Here's how the part is built. I have some questions about the finished solid (model axes, mm). Face numbers are marked on the shaded views. A direction names the side the tool comes from. Round coordinates to 2 decimals unless told otherwise and drop trailing zeros. Order: outer loops, then holes, each group sorted by start corner. A loop starts at its lowest first (then second) coordinate and runs counter-clockwise, first axis right, second up. Notation, with made-up numbers: (-21.5, 87) -> (-16.5, 87) arc R36 ccw to (-16.5, 125) -> close; hole circle Ø1 at (-39.75, 75). An arc over 180 degrees is marked (long way). Use a Markdown table: item, result. Add a question column.
(1) I want a section at A-A, the plane z = -54.25. Please give me the cut outline in (x, y) (3 decimals).
(2) If I drill on probe 1 along Z at (x, y) = (-3.25, -21.75); probe 2 along X at (y, z) = (-15.5, -49); probe 3 along X at (y, z) = (-19, -40.75), over which ranges is the centre line in solid material (lowest first)?
(3) Thinking about a two-plate mould opening in Z: for the marked faces 4, 5 and 6, which applies, pulls with the +Z half, pulls with the -Z half, needs draft (parallel to the pull), parting line crosses it, or undercut?
(4) On a 3-axis mill with a long thin cutter (end or side, diameter ignored), from which of +Z, -Z, +X, -X, +Y, -Y can I reach the whole of each face in a straight line? I mean the marked faces 1, 2 and 3. Say none if no direction works.
(5) I want a section at B-B, the plane x = -2.5. Please give me the cut outline in (y, z).
(6) I want a section at C-C, the plane y = -23.75. Please give me the cut outline in (x, z) (3 decimals), then the cut area to 3 significant figures.
(7) I want a section at D-D, the plane z = -51. Please give me the cut outline in (x, y) (3 decimals).
(8) I'm going to push flat-ended pins straight in: P1, Ø2.5, axis at x = 0, z = -48.5, coming from the +Y side; P2, Ø2.5, axis at x = -7, z = -48, coming from the +Y side; P3, Ø2, axis at y = -18.5, z = -54, coming from the -X side (3 decimals); P4, Ø2.5, axis at x = -3.375, z = -50, coming from the +Y side. Where does each tip first touch, or does it pass through?
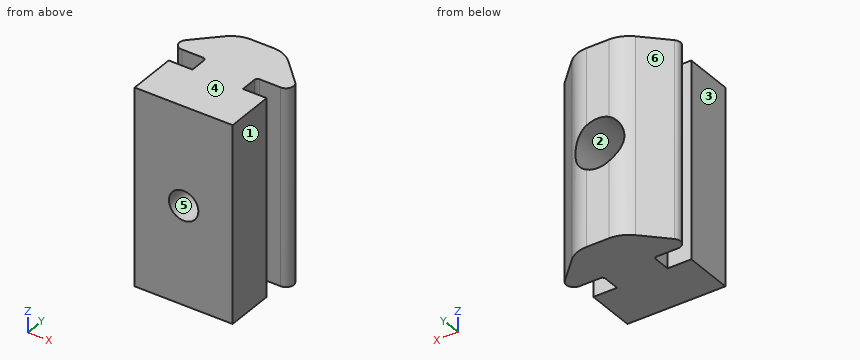
from build123d import *

# Parameters (mm, degrees)
F1_DEPTH = 60
F2_R     = 1.5
F3_DEPTH = 25
F4_R     = 2.5
F5_R     = 2.5
F6_DEPTH = 5
F7_DEPTH = 40


with BuildPart() as f1:
    # F0 (on Top) → F1 (new body)
    with BuildSketch(Plane.XY):
        with BuildLine():
            Line((-0.8000000172, -20.2), (-0.8000000172, -19.2))
            Line((-0.8, -19.2), (-0.8, -18.5000007629))
            ThreePointArc((-0.8, -18.5000007629), (-0.7121320729, -18.2878687671), (-0.5000001089, -18.2000007629))
            Line((-0.5000001089, -18.2000007629), (1.6691214738, -18.1999999754))
            ThreePointArc((1.6691214738, -18.1999999754), (2.3897472802, -17.7184929218), (2.2206644799, -16.868456686))
            Line((2.2206644799, -16.868456686), (-0.1191125495, -14.5286796566))
            ThreePointArc((-0.1191125495, -14.5286796566), (-1.0923825989, -13.8783614014), (-2.2404328993, -13.6500000001))
            Line((-2.2404328993, -13.6500000001), (-4.5095671179, -13.6500000049))
            ThreePointArc((-4.5095671179, -13.6500000049), (-5.6576174116, -13.8783614085), (-6.6308874552, -14.5286796613))
            Line((-6.6308874552, -14.5286796613), (-8.970664486, -16.8684566921))
            ThreePointArc((-8.970664486, -16.8684566921), (-9.1397472858, -17.7184929288), (-8.4191214777, -18.1999999814))
            Line((-8.4191214777, -18.1999999814), (-6.2499998919, -18.2000007629))
            ThreePointArc((-6.2499998919, -18.2000007629), (-6.0378679274, -18.2878687668), (-5.95, -18.5000007629))
            Line((-5.95, -18.5000007629), (-5.95, -19.2))
            Line((-5.95, -19.2), (-5.95, -20.2))
            Line((-5.95, -20.2), (-8.3750000086, -20.2))
            Line((-8.3750000086, -20.2), (-8.3750000086, -25.2))
            Line((-8.3750000086, -25.2), (-3.3750000086, -25.2))
            Line((-3.3750000086, -25.2), (1.6249999914, -25.2))
            Line((1.6249999914, -25.2), (1.6249999914, -20.2))
            Line((1.6249999914, -20.2), (-0.8000000172, -20.2))
        make_face()
    extrude(amount=-F1_DEPTH)

    # F2 (on face) → F3 (cut)
    with BuildSketch(Plane.XZ.offset(25.2)):
        with Locations((-3.3750000086, -50)):
            Circle(F2_R)
        with Locations((-3.3750000086, -30)):
            Circle(F2_R)
        with Locations((-3.3750000086, -10)):
            Circle(F2_R)
    extrude(amount=-F3_DEPTH, mode=Mode.SUBTRACT)

    # F4 (on face) + F5 (on face) → F6 (cut)
    with BuildSketch(Plane(origin=(2.85e-08, -13.6499999955, 0), x_dir=(-1, -2.1e-09, 0), z_dir=(-2.1e-09, 1, 0))):
        with Locations((3.3750000371, -10)):
            Circle(F4_R)
        with Locations((3.3750000371, -30)):
            Circle(F4_R)
    with BuildSketch(Plane(origin=(2.85e-08, -13.6499999955, 0), x_dir=(-1, -2.1e-09, 0), z_dir=(-2.1e-09, 1, 0))):
        with Locations((3.3750000371, -50)):
            Circle(F5_R)
    extrude(amount=-F6_DEPTH, mode=Mode.SUBTRACT)

    # F7 (cut): a face of the model
    f7_faces = [f1.faces().sort_by_distance(p)[0] for p in [
        (-3.3750000055, -19.7568505706, 0),
    ]]
    extrude(f7_faces, amount=-F7_DEPTH, mode=Mode.SUBTRACT)


solid = f1.part
Taken from the geometry:
| question | item | result |
|---|---|---|
| 1 | outline | (-8.971, -16.868) arc R0.78 ccw to (-8.419, -18.2) -> (-6.25, -18.2) arc R0.3 cw to (-5.95, -18.5) -> (-5.95, -20.2) -> (-8.375, -20.2) -> (-8.375, -25.2) -> (1.625, -25.2) -> (1.625, -20.2) -> (-0.8, -20.2) -> (-0.8, -18.5) arc R0.3 cw to (-0.5, -18.2) -> (1.669, -18.2) arc R0.78 ccw to (2.221, -16.868) -> (-0.119, -14.529) arc R3 ccw to (-2.24, -13.65) -> (-4.51, -13.65) arc R3 ccw to (-6.631, -14.529) -> close |
| 2 | probe 1 | z = -60 to -51.49, -48.51 to -40 |
| 2 | probe 2 | x = -7.6 to -5.67, -1.08 to 0.85 |
| 2 | probe 3 | x = -5.95 to -0.8 |
| 3 | face 4 | pulls with the +Z half |
| 3 | face 5 | undercut |
| 3 | face 6 | needs draft |
| 4 | face 1 | +Z, -Z, +X, -Y |
| 4 | face 2 | +Y |
| 4 | face 3 | +Z, -Z, -X, -Y |
| 5 | outline | (-25.2, -60) -> (-13.65, -60) -> (-13.65, -52.34) -> (-18.65, -52.34) -> (-18.65, -51.22) -> (-25.2, -51.22) -> close; (-25.2, -48.78) -> (-18.65, -48.78) -> (-18.65, -47.66) -> (-13.65, -47.66) -> (-13.65, -40) -> (-25.2, -40) -> close |
| 6 | outline | (-8.375, -60) -> (1.625, -60) -> (1.625, -40) -> (-8.375, -40) -> close; hole circle Ø3 at (-3.375, -50) |
| 6 | area | 193 mm2 |
| 7 | outline | (-8.971, -16.868) arc R0.78 ccw to (-8.419, -18.2) -> (-6.25, -18.2) arc R0.3 cw to (-5.95, -18.5) -> (-5.95, -20.2) -> (-8.375, -20.2) -> (-8.375, -25.2) -> (-4.493, -25.2) -> (-4.493, -18.65) -> (-5.666, -18.65) -> (-5.666, -13.882) arc R3 ccw to (-6.631, -14.529) -> close; (-2.257, -25.2) -> (1.625, -25.2) -> (1.625, -20.2) -> (-0.8, -20.2) -> (-0.8, -18.5) arc R0.3 cw to (-0.5, -18.2) -> (1.669, -18.2) arc R0.78 ccw to (2.221, -16.868) -> (-0.119, -14.529) arc R3 ccw to (-1.084, -13.882) -> (-1.084, -18.65) -> (-2.257, -18.65) -> close |
| 8 | P1 | stops at y = -13.82 |
| 8 | P2 | stops at y = -13.92 |
| 8 | P3 | stops at x = -9.195 |
| 8 | P4 | passes through |
